Job drawing, mm, ordinate dimensions from the low corner. One solid piece. Coordinates: 2 decimals unless noted, no trailing zeros. Write each loop counter-clockwise with the first axis right and the second up, starting at its lowest first coordinate (ties: lowest second). Pieces come first, ordered by that corner, then holes.
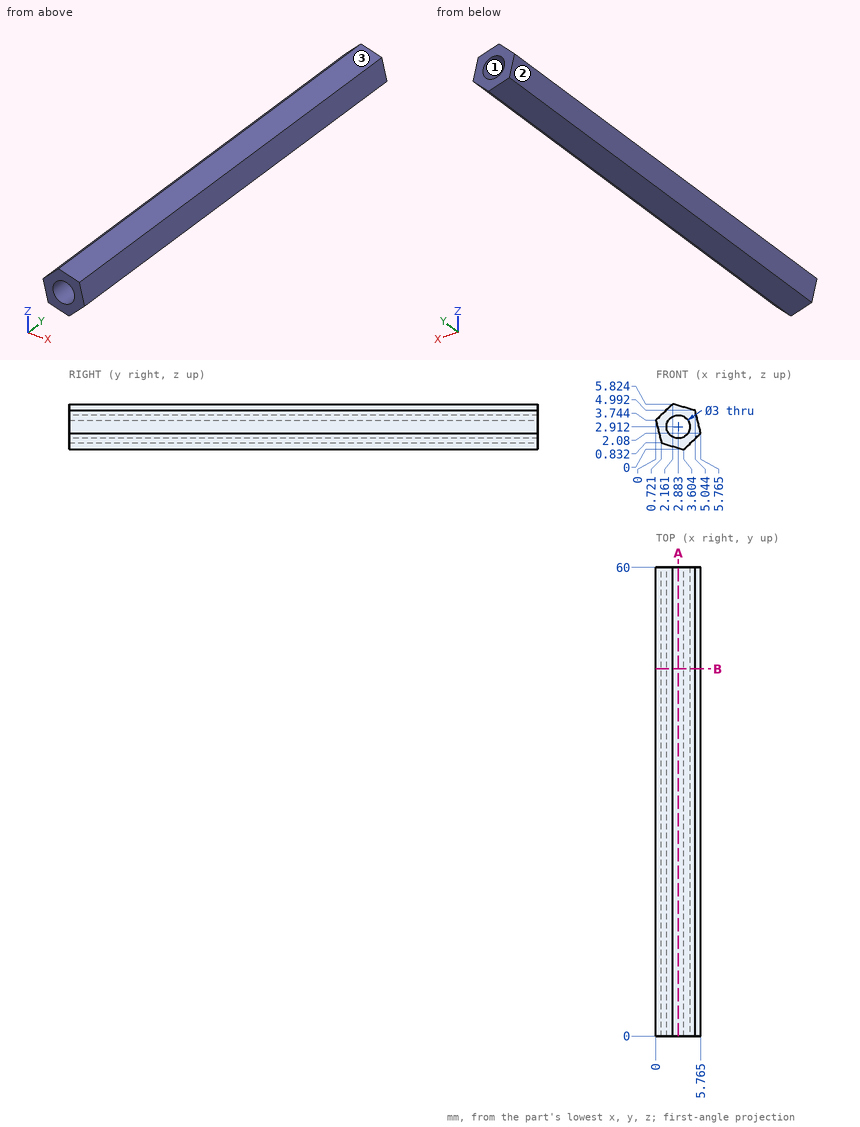
1. Saw through at B-B on y = 47. List the corners of the cut face in (x, z) (1 decimal).
Computed values:
outline: (0, 3.7) - (0.7, 0.8) - (3.6, 0) - (5.8, 2.1) - (5, 5) - (2.2, 5.8) - close; hole circle Ø3 at (2.9, 2.9)
2. Flat gauge pin, fed straight in: pin 1 (2.5 mm diameter, centred on x = 2.88, z = 2.91, fed in from +Y). Where does the tip first touch, or does it go through?
Computed values:
pin 1: passes through
3. Mould opens along X. For the marked faces 1, 2 and 3 say: +X half, -X half, draft (parallel to the pull), parting line (faces both ways), or undercut.
Computed values:
face 1: undercut
face 2: -X half
face 3: +X half
4. Probe line 1 along Z through (x, y) = (2, 54) (1 decimal); line 2 along Z through (x, y) = (3.2, 49.5) (1 decimal); line 3 along X through (y, z) = (53, 2.1) (1 decimal). List the from-to ranges inside material, lowest first.
Computed values:
line 1: z = 0.5 to 1.7, 4.1 to 5.7
line 2: z = 0.1 to 1.4, 4.4 to 5.5
line 3: x = 0.4 to 1.6, 4.1 to 5.8
5. Saw through at A-A on x = 2.9. List the corners of the cut face in (y, z).
Computed values:
outline: (0, 0.2) - (60, 0.2) - (60, 1.41) - (0, 1.41) - close; (0, 4.41) - (60, 4.41) - (60, 5.61) - (0, 5.61) - close
